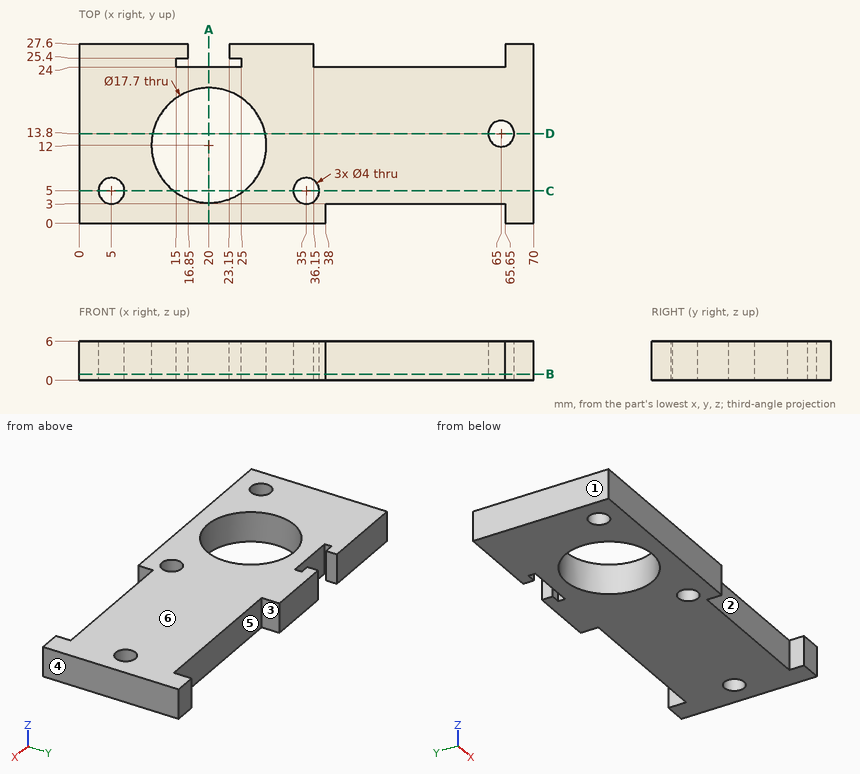
Can you work these out from the drawing? Everything is in mm from the part's minimum corner. A direction names the side the tool comes from. Coordinates: 2 decimals unless noted, no trailing zeros. Loops run counter-clockwise (first coordinate to the right, second up) from the corner with the lowest first, then second, coordinate; pieces in that order, holes last. Notation, with made-up numbers: (47, 14.25) - (90, 14.25) arc R24 ccw to (90, 26.25) - close; hole circle Ø8 at (69, 73). An arc over 180 degrees is marked (long way). Put each result on its own line as item: value. Start each with the question number.
Item 1: Suppose I cut it at A-A (x = 20). Please give me the cut outline in (y, z), and give its area (3 significant figures).
Item 2: If I drill on line 1 along Y through (x, z) = (20, 2.1); line 2 along Y through (x, z) = (65, 4); line 3 along X through (y, z) = (24.25, 2.85), over which ranges is the centre line in solid material (lowest first)?
Item 3: For pin 1 (3 mm diameter, centred on y = 21.5, z = 0.5, fed in from -X); pin 2 (6 mm diameter, centred on x = 22.5, y = 16, fed in from -Z); pin 3 (1.8 mm diameter, centred on x = 21, z = 2.5, fed in from +Y), each with a flat end and sliding along its axis, tell me the tip position at first contact or that it passes through.
Item 4: Suppose I cut it at B-B (z = 0.95). Please give me the cut outline in (x, y).
Item 5: If we mould it in two halves opening along X, with no side actions, what happens to the marked faces 4, 5 and 6? For each: +X half, -X half, draft (parallel to the pull), parting line (faces both ways), or undercut.
Item 6: Suppose I cut it at C-C (y = 5). Please give me the cut outline in (x, z), and give its area (3 significant figures).
Item 7: Suppose I cut it at D-D (y = 13.8). Please give me the cut outline in (x, z), and give its area (3 significant figures).
Item 8: Which directions (+Z, -Z, +X, -X, +Y, -Y) give clear straight access to the entire face, cutting with the end or side of a thin tool? Please do the marked faces 1, 2 and 3.
Here are the results:
1. outline: (0, 0) - (3.15, 0) - (3.15, 6) - (0, 6) - close; (20.85, 0) - (24, 0) - (24, 6) - (20.85, 6) - close
1. area: 37.8 mm²
2. line 1: 0 to 3.15, 20.85 to 24
2. line 2: 3 to 11.8, 15.8 to 24
2. line 3: 0 to 15, 25 to 36.15, 65.65 to 70
3. pin 1: x = 0
3. pin 2: through
3. pin 3: y = 24
4. outline: (0, 0) - (38, 0) - (38, 3) - (65.65, 3) - (65.65, 0) - (70, 0) - (70, 27.6) - (65.65, 27.6) - (65.65, 24) - (36.15, 24) - (36.15, 27.6) - (23.15, 27.6) - (23.15, 25.4) - (25, 25.4) - (25, 24) - (15, 24) - (15, 25.4) - (16.85, 25.4) - (16.85, 27.6) - (0, 27.6) - close; hole circle Ø4 at (5, 5); hole circle Ø17.7 at (20, 12); hole circle Ø4 at (35, 5); hole circle Ø4 at (65, 13.8)
5. face 4: +X half
5. face 5: undercut
5. face 6: draft
6. outline: (0, 0) - (3, 0) - (3, 6) - (0, 6) - close; (7, 0) - (14.58, 0) - (14.58, 6) - (7, 6) - close; (25.42, 0) - (33, 0) - (33, 6) - (25.42, 6) - close; (37, 0) - (70, 0) - (70, 6) - (37, 6) - close
6. area: 307 mm²
7. outline: (0, 0) - (11.33, 0) - (11.33, 6) - (0, 6) - close; (28.67, 0) - (63, 0) - (63, 6) - (28.67, 6) - close; (67, 0) - (70, 0) - (70, 6) - (67, 6) - close
7. area: 292 mm²
8. face 1: +Z, -Z, -X, +Y, -Y
8. face 2: +Z, -Z, -Y
8. face 3: +Z, -Z, +Y
